from build123d import *

# Parameters (mm, degrees)
F2_R = 0.2


with BuildPart() as f1:
    # F0 (on Front) → F1 (revolve)
    with BuildSketch(Plane.XZ):
        with BuildLine():
            Line((10.435, 14.422704), (0, 14.422704))
            Line((0, 14.422704), (0, 10.294014))
            Line((0, 10.294014), (3.405, 10.294014))
            Line((3.405, 10.294014), (4.58817, 6.672704))
            Line((4.58817, 6.672704), (6.81, 6.672704))
            Line((6.81, 6.672704), (6.81, 7.497758))
            ThreePointArc((6.81, 7.497758), (5.410053, 8.897704), (6.81, 10.297651))
            Line((6.81, 10.297651), (6.81, 11.122704))
            Line((6.81, 11.122704), (10.435, 11.122704))
            Line((10.435, 11.122704), (10.435, 14.422704))
        make_face()
    revolve(axis=Axis((0, 0, 6.85568), (0, 0, -1)))

    # F2
    f2_edges = [f1.edges().sort_by_distance(p)[0] for p in [
        (-10.435, 0, 14.422704),
    ]]
    fillet(f2_edges, radius=F2_R)


solid = f1.part
Can you work these out from the model? Positions are in its coordinate system, mm. A direction names the side the tool comes from. Coordinates: 2 decimals unless noted, no trailing zeros. Loops run counter-clockwise (first coordinate to the right, second up) from the corner with the lowest first, then second, coordinate; pieces in that order, holes last. Notation, with made-up numbers: M 51.25,-18 L 81.25,-18 A13 cw 81.25,-5 Z; hole C -10.75,-31.75 d5. An arc over 180 degrees is marked long. Return JSON: item names as keys, results as strings. Group by question number.
Item 1: If I drill on L1, parallel to Y at x = 0.25, z = 11; L2, parallel to Z at x = -5.25, y = 3.25; L3, parallel to X at y = -0.5, z = 8.75, over which ranges is the centre line in solid material (lowest first)? Write a range as from..to.
Item 2: On a 3-axis mill with a long thin cutter (end or side, diameter ignored), from which of +Z, -Z, +X, -X, +Y, -Y can I reach the whole of each face in a straight line? I mean faces 1 (the cylindrical face through (3.142, 6.042, 7.091)), 2 (the flat face through (0, -5, 6.673)). Say none if no direction works.
Item 3: Imagine slicing it at A-A (x = 0). Please give me the cut outline in (y, z) (3 decimals), and give its area (3 significant figures).
Item 4: I'm going to push flat-ended pins straight in: pin 1 Ø2 at (x, z) = (2.5, 11.5) entering from -Y; pin 2 Ø2 at (x, y) = (0, -0.5) entering from -Z. Where does each tip first touch, or does it pass through?
Item 5: Imagine slicing it at C-C (z = 9.5). Please give me the cut outline in (x, y).
Item 6: Thinking about a two-plate mould opening in Y: for faces 3 (the conical face through (1.67, 3.2, 9.67)), 4 (the flat face through (0, 7, 11.123)), 5 (the flat face through (0, 0, 10.294)), 6 (the cylindrical face through (4.815, 9.258, 12.694)), which applies, released by +Y, released by -Y, zero draft, split by the parting line, or undercut?
Verdict:
{
 "1": {"L1": "y = -6.81..6.81", "L2": "z = 6.67..7.65, 10.15..14.42", "L3": "x = -5.39..-3.88, 3.88..5.39"},
 "2": {"face 1": "-Z", "face 2": "-Z, +X, -X, +Y, -Y"},
 "3": {"outline": "M -10.435,11.123 L -6.81,11.123 L -6.81,10.298 A1.4 cw -6.81,7.498 L -6.81,6.673 L -4.588,6.673 L -3.405,10.294 L 3.405,10.294 L 4.588,6.673 L 6.81,6.673 L 6.81,7.498 A1.4 cw 6.81,10.298 L 6.81,11.123 L 10.435,11.123 L 10.435,14.223 A0.2 ccw 10.235,14.423 L -10.235,14.423 A0.2 ccw -10.435,14.223 Z", "area": "94.4 mm^2"},
 "4": {"pin 1": "stops at y = -10.33", "pin 2": "stops at z = 10.29"},
 "5": {"outline": "C 0,0 d11.09; hole C 0,0 d7.33"},
 "6": {"face 3": "undercut", "face 4": "zero draft", "face 5": "undercut", "face 6": "split by the parting line"}
}
